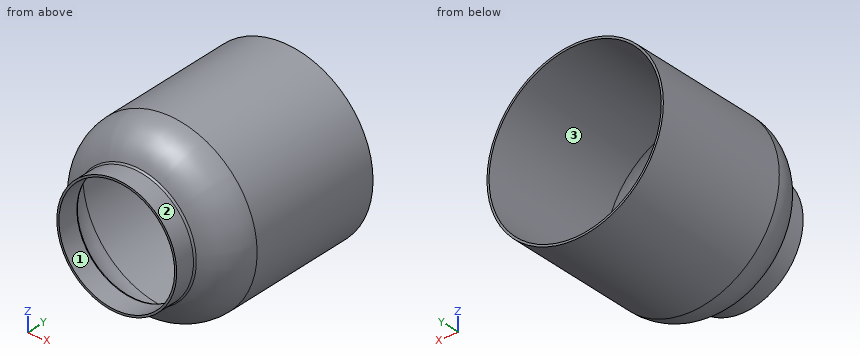
```python
from build123d import *


with BuildPart() as part:
    # Çizim1 → Döndür1 (revolve)
    with BuildSketch(Plane.XY, mode=Mode.PRIVATE) as d_nd_r1_sk:
        with BuildLine():
            Line((-62.5, 208.714063436), (-62.5, 108.714063436))
            ThreePointArc((-62.5, 108.714063436), (-57.140269015, 91.600994078), (-42.976190476, 80.602687925))
            ThreePointArc((-42.976190476, 80.602687925), (-42.267986549, 80.052772618), (-42, 79.19711915))
            Line((-42, 79.19711915), (-42, 63.714063436))
            Line((-42, 63.714063436), (-43.5, 63.714063436))
            Line((-43.5, 63.714063436), (-43.5, 78.173107328))
            ThreePointArc((-43.5, 78.173107328), (-43.754553749, 79.009087972), (-44.431818182, 79.561332606))
            ThreePointArc((-44.431818182, 79.561332606), (-58.654371267, 91.158469922), (-64, 108.714063436))
            Line((-64, 108.714063436), (-64, 208.714063436))
            Line((-64, 208.714063436), (-62.5, 208.714063436))
        make_face()
    revolve(d_nd_r1_sk.sketch.rotate(Axis((0, 0, 0), (0, 1, 0)), 270), axis=Axis((0, 0, 0), (0, 1, 0)))


solid = part.part
```
Source: CAD feature listing. Evaluate the final solid. Frame: model axes, mm. Face numbers are marked on the shaded views. Give positions to 0.01 mm unless a question says otherwise; leave off trailing zeros. Loops run counter-clockwise (first coordinate to the right, second up) from the corner with the lowest first, then second, coordinate; pieces in that order, holes last. Notation, with made-up numbers: (74, 4) - (123, 4) arc R24 cw to (123, 32) - close; hole circle Ø9 at (82, 78). An arc over 180 degrees is marked (long way). Use CSV: the item, a comma, the result in double quotes.
1) Cut plane B-B (z = 0). Output: boundary loops of the cut face in (x, y), and give its area (3 significant figures).
Worked out:
outline,"(-64, 108.71) arc R31.5 ccw to (-44.43, 79.56) arc R1.5 cw to (-43.5, 78.17) - (-43.5, 63.71) - (-42, 63.71) - (-42, 79.2) arc R1.5 ccw to (-42.98, 80.6) arc R30 cw to (-62.5, 108.71) - (-62.5, 208.71) - (-64, 208.71) - close; (42, 63.71) - (43.5, 63.71) - (43.5, 78.17) arc R1.5 cw to (44.43, 79.56) arc R31.5 ccw to (64, 108.71) - (64, 208.71) - (62.5, 208.71) - (62.5, 108.71) arc R30 cw to (42.98, 80.6) arc R1.5 ccw to (42, 79.2) - close"
area,"462 mm^2"
2) Cut plane C-C (y = 133). Output: boundary loops of the cut face in (x, z), and give its area (3 significant figures).
Worked out:
outline,"circle Ø128 at (0, 0); hole circle Ø125 at (0, 0)"
area,"596 mm^2"
3) Line query: line 1 (X direction, y = 70.75, z = 0); line 2 (X direction, y = 146, z = 0); line 3 (Z direction, x = -23, y = 141). Output: solid intervals per line, ascending.
Worked out:
line 1,"x = -43.5 to -42, 42 to 43.5"
line 2,"x = -64 to -62.5, 62.5 to 64"
line 3,"z = -59.72 to -58.11, 58.11 to 59.72"
4) Pin query (flat end, axial travel): P1, Ø1, axis at x = 33.5, y = 148, coming from the -Z side; P2, Ø10, axis at x = -19, y = 138, coming from the -Z side; P3, Ø10, axis at x = 49, z = 14, coming from the +Y side. Return the tip coordinate at first contact, or that it passes through.
Worked out:
P1,"stops at z = -54.84"
P2,"stops at z = -62.45"
P3,"stops at y = 90.02"
5) Cut plane A-A (x = 0). Output: boundary loops of the cut face in (y, z).
Worked out:
outline,"(63.71, -43.5) - (78.17, -43.5) arc R1.5 cw to (79.56, -44.43) arc R31.5 ccw to (108.71, -64) - (208.71, -64) - (208.71, -62.5) - (108.71, -62.5) arc R30 cw to (80.6, -42.98) arc R1.5 ccw to (79.2, -42) - (63.71, -42) - close; (63.71, 42) - (79.2, 42) arc R1.5 ccw to (80.6, 42.98) arc R30 cw to (108.71, 62.5) - (208.71, 62.5) - (208.71, 64) - (108.71, 64) arc R31.5 ccw to (79.56, 44.43) arc R1.5 cw to (78.17, 43.5) - (63.71, 43.5) - close"
6) Mould query, pull axis X, two halves, no side actions, for the marked faces 1, 2 and 3. Classes: +X half, -X half, draft (parallel to the pull), parting line (faces both ways), or undercut.
Worked out:
face 1,"undercut"
face 2,"parting line"
face 3,"undercut"
